Can you work these out from the model? Positions are in its coordinate system, mm. Face numbers are marked on the shaded views. A direction names the side the tool comes from. Round coordinates to 2 decimals unless told otherwise and drop trailing zeros. Loops run counter-clockwise (first coordinate to the right, second up) from the corner with the lowest first, then second, coordinate; pieces in that order, holes last.
from build123d import *

# Parameters (mm, degrees)
F0_W      = 31.75
F0_H      = 31.75
F0_R      = 4.2545
F1_DEPTH  = 38.1
F2_R      = 1.27
F3_DEPTH  = 76.2
F2_R_2    = 3.175
F4_DEPTH  = 6.35
F6_W      = 31.75
F6_H      = 31.75
F6_W_2    = 25.4
F6_H_2    = 25.4
F7_DEPTH  = 9.525
F8_DEPTH  = 101.6
F9_W      = 3.175
F9_H      = 1.27
F9_W_2    = 1.27
F9_H_2    = 12.7
F10_DEPTH = 25.4
F11_W     = 3.175
F11_H     = 12.7
F11_W_2   = 1.016
F11_W_3   = 4.191
F12_DEPTH = 6.35
F13_SIZE  = 1.01599
F14_W     = 12.7
F14_H     = 12.7
F14_R     = 4.2545
F15_DEPTH = 12.7
F16_SIZE  = 4.1275


# Not quite as in the source:
# - a fillet or chamfer is up to 0.001 mm smaller than in the source, because OpenCascade refuses the exact size


with BuildPart() as f1:
    # F0 (on Top) → F1 (new body)
    with BuildSketch(Plane.XY):
        Rectangle(F0_W, F0_H)
        Circle(F0_R, mode=Mode.SUBTRACT)
    extrude(amount=F1_DEPTH)

    # F2 (on face) → F3 (cut)
    with BuildSketch(Plane.XZ.offset(15.875)):
        with Locations((0, 3.302)):
            Circle(F2_R)
    extrude(amount=-F3_DEPTH, mode=Mode.SUBTRACT)

    # F2 (on face) → F4 (cut)
    with BuildSketch(Plane.XZ.offset(15.875)):
        with Locations((0, 3.302)):
            Circle(F2_R_2)
        with Locations((0, 3.302)):
            Circle(F2_R, mode=Mode.SUBTRACT)
    extrude(amount=-F4_DEPTH, mode=Mode.SUBTRACT)

    # F6 (on face) → F7 (cut)
    with BuildSketch(Plane.XY.offset(38.1)):
        Rectangle(F6_W, F6_H)
        Rectangle(F6_W_2, F6_H_2, mode=Mode.SUBTRACT)
    extrude(amount=-F7_DEPTH, mode=Mode.SUBTRACT)

    # F5 (on face) → F8 (cut)
    with BuildSketch(Plane(origin=(0, 0, 0), x_dir=(1, 0, 0), z_dir=(0, 0, -1))):
        with BuildLine():
            Line((15.875, -15.875), (15.875, 0))
            ThreePointArc((15.875, 0), (11.2253201706, -11.2253201321), (5.44e-08, -15.875))
            Line((5.44e-08, -15.875), (15.875, -15.875))
        make_face()
        with BuildLine():
            Line((-15.875, -15.875), (5.44e-08, -15.875))
            ThreePointArc((5.44e-08, -15.875), (-11.2253201321, -11.2253201706), (-15.875, 0))
            Line((-15.875, 0), (-15.875, -15.875))
        make_face()
        with BuildLine():
            ThreePointArc((-15.875, 0), (-11.2253201513, 11.2253201513), (0, 15.875))
            Line((0, 15.875), (-15.875, 15.875))
            Line((-15.875, 15.875), (-15.875, 0))
        make_face()
        with BuildLine():
            ThreePointArc((0, 15.875), (11.2253201513, 11.2253201513), (15.875, 0))
            Line((15.875, 0), (15.875, 15.875))
            Line((15.875, 15.875), (0, 15.875))
        make_face()
    extrude(amount=-F8_DEPTH, mode=Mode.SUBTRACT)

    # F9 (on face) → F10 (cut)
    with BuildSketch(Plane.XY.offset(38.1)):
        with Locations((-14.2875, 6.985)):
            Rectangle(F9_W, F9_H)
        with Locations((-11.1125, 6.985)):
            Rectangle(F9_W, F9_H)
        with Locations((-8.89, 6.985)):
            Rectangle(F9_W_2, F9_H)
        with Locations((-8.89, 0)):
            Rectangle(F9_W_2, F9_H_2)
        with Locations((-8.89, -6.985)):
            Rectangle(F9_W_2, F9_H)
        with Locations((-11.1125, -6.985)):
            Rectangle(F9_W, F9_H)
        with Locations((-14.2875, -6.985)):
            Rectangle(F9_W, F9_H)
        with Locations((14.2875, 6.985)):
            Rectangle(F9_W, F9_H)
        with Locations((11.1125, 6.985)):
            Rectangle(F9_W, F9_H)
        with Locations((8.89, 6.985)):
            Rectangle(F9_W_2, F9_H)
        with Locations((8.89, 0)):
            Rectangle(F9_W_2, F9_H_2)
        with Locations((8.89, -6.985)):
            Rectangle(F9_W_2, F9_H)
        with Locations((11.1125, -6.985)):
            Rectangle(F9_W, F9_H)
        with Locations((14.2875, -6.985)):
            Rectangle(F9_W, F9_H)
    extrude(amount=-F10_DEPTH, mode=Mode.SUBTRACT)

    # F11 (on face) → F12 (join)
    with BuildSketch(Plane.XY.offset(38.1)):
        with Locations((11.1125, 0)):
            Rectangle(F11_W, F11_H)
        with Locations((13.208, 0)):
            Rectangle(F11_W_2, F11_H)
        with Locations((-11.6205, 0)):
            Rectangle(F11_W_3, F11_H)
    extrude(amount=F12_DEPTH)

    # F13 (size 1.016 in the source; OpenCascade refuses exactly that, so slightly less here)
    f13_edges = [f1.edges().sort_by_distance(p)[0] for p in [
        (13.716, 0, 38.1),
        (-13.716, 0, 38.1),
    ]]
    chamfer(f13_edges, length=F13_SIZE)

    # F14 (on face) → F15 (join)
    with BuildSketch(Plane.XY.offset(38.1)):
        Rectangle(F14_W, F14_H)
        Circle(F14_R, mode=Mode.SUBTRACT)
        Circle(F14_R)
    extrude(amount=-F15_DEPTH)

    # F16
    f16_edges = [f1.edges().sort_by_distance(p)[0] for p in [
        (-4.2545, 0, 25.4),
    ]]
    chamfer(f16_edges, length=F16_SIZE)


solid = f1.part
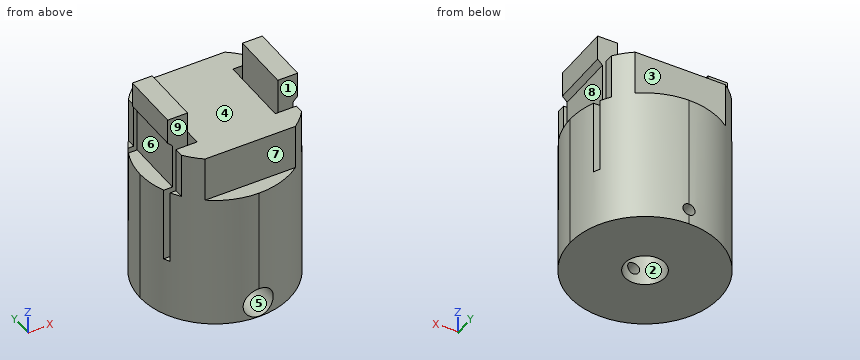
(1) If we mould it in two halves opening along Y, with no side actions, what happens to the marked faces 1, 2, 3 and 4? For each: released by +Y, released by -Y, zero draft, split by the parting line, or undercut.
Worked answers:
face 1: undercut
face 2: undercut
face 3: released by +Y
face 4: zero draft
(2) If we section it at C-C, the plane x = 12: List the corners of the cut face in (y, z) for me, then the cut area to 3 significant figures.
Worked answers:
outline: (-10.39, 0) - (10.39, 0) - (10.39, 38.1) - (7.62, 38.1) - (7.62, 12.7) - (6.35, 12.7) - (6.35, 44.45) - (-6.35, 44.45) - (-6.35, 12.7) - (-7.62, 12.7) - (-7.62, 38.1) - (-10.39, 38.1) - close
area: 808 mm2
(3) If we section it at A-A, the plane z = 26.5: List the corners of the cut face in (x, y) for me (3 decimals).
Worked answers:
outline: (-14.55, -6.35) - (-9.525, -6.35) - (-9.525, 6.35) - (-14.55, 6.35) arc R15.875 ccw to start; (-13.927, -7.62) arc R15.875 ccw to (13.927, -7.62) - (8.255, -7.62) - (8.255, 7.62) - (13.927, 7.62) arc R15.875 ccw to (-13.927, 7.62) - (-8.255, 7.62) - (-8.255, -7.62) - close; (9.525, -6.35) - (14.55, -6.35) arc R15.875 ccw to (14.55, 6.35) - (9.525, 6.35) - close
(4) Will these pins go through, and if not, where does the flat tip stop? P1, Ø12, axis at y = -10.5, z = 36, coming from the -X side; P2, Ø3.5, axis at x = 0, z = 3.302, coming from the -Y side (3 decimals); P3, Ø1, axis at x = 13.5, y = 9, coming from the +Z side (3 decimals).
Worked answers:
P1: stops at x = -13.72
P2: stops at y = -9.525
P3: stops at z = 28.575
(5) If I drill on line 1 (X direction, y = -2.5, z = 41) (3 decimals); line 2 (Y direction, x = 13, z = 28); line 3 (X direction, y = 1, z = 14) (3 decimals), over which ranges is the centre line in solid material (lowest first)?
Worked answers:
line 1: x = -13.716 to -9.525, 9.525 to 13.716
line 2: y = -9.11 to -7.62, -6.35 to 6.35, 7.62 to 9.11
line 3: x = -15.843 to -9.525, -8.255 to -4.135, 4.135 to 8.255, 9.525 to 15.843
(6) For the marked faces 5, 6, 7, 8 and 9, which set-ups out of +Z, -Z, +X, -X, +Y, -Y let a thin tool reach every point of the face, with its end or its side?
Worked answers:
face 5: -Y
face 6: -X, +Y, -Y
face 7: +Z, +X, -X, -Y
face 8: +X, +Y, -Y
face 9: +Z, -X
